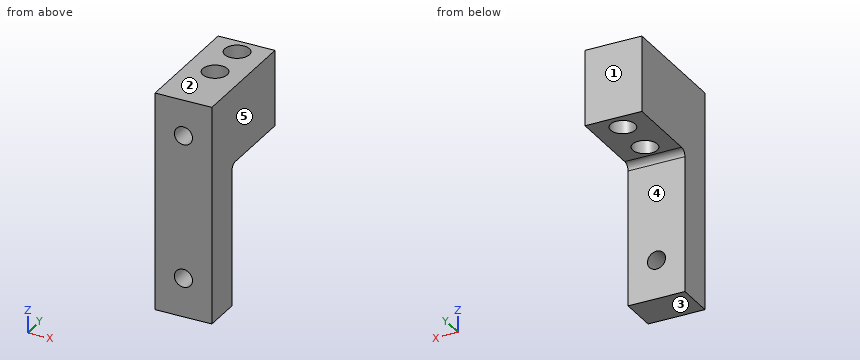
```python
from build123d import *

# Parameters (mm, degrees)
SKETCH1_W                 = 18.25
SKETCH1_H                 = 10
BOSS_EXTRUDE1_DEPTH       = 4.7625
F_1_64_TAPPED_HOLE1_D     = 1.5113
F_1_64_TAPPED_HOLE1_DEPTH = 3.5
F_1_64_TAPPED_HOLE1_TIP   = 0.454040327
SKETCH5_W                 = 11.9
SKETCH5_H                 = 6.825
CUT_EXTRUDE2_DEPTH        = 10
FILLET1_R                 = 0.5334
SKETCH2_R                 = 1.03
CUT_EXTRUDE1_DEPTH        = 20.512660153


with BuildPart() as part:
    # Sketch1 → Boss-Extrude1 (new body)
    with BuildSketch(Plane(origin=(0, 0, 0), x_dir=(0, 0, -1), z_dir=(1, 0, 0))):
        Rectangle(SKETCH1_W, SKETCH1_H)
    extrude(amount=BOSS_EXTRUDE1_DEPTH)

    # #1-64 Tapped Hole1
    with Locations(Plane(origin=(0, -5, 0), x_dir=(-1, 0, 0), z_dir=(0, -1, 0))):
        with Locations((-2.38125, -6.125), (-2.38125, 5.875)):
            Hole(F_1_64_TAPPED_HOLE1_D / 2, depth=F_1_64_TAPPED_HOLE1_DEPTH)
            with Locations((0, 0, -(F_1_64_TAPPED_HOLE1_DEPTH + F_1_64_TAPPED_HOLE1_TIP / 2))):  # 118° drill point
                Cone(0, F_1_64_TAPPED_HOLE1_D / 2, F_1_64_TAPPED_HOLE1_TIP, mode=Mode.SUBTRACT)

    # Sketch5 → Cut-Extrude2 (cut)
    with BuildSketch(Plane(origin=(4.7625, 0, 0), x_dir=(0, 0, -1), z_dir=(1, 0, 0))):
        with Locations((3.175, 1.5875)):
            Rectangle(SKETCH5_W, SKETCH5_H)
    extrude(amount=-CUT_EXTRUDE2_DEPTH, mode=Mode.SUBTRACT)

    # Fillet1
    fillet1_edges = [part.edges().sort_by_distance(p)[0] for p in [
        (2.38125, -1.825, 2.775),
    ]]
    fillet(fillet1_edges, radius=FILLET1_R)

    # Sketch2 → Cut-Extrude1 (cut, through all)
    with BuildSketch(Plane(origin=(0, 0, -9.125), x_dir=(-1, 0, 0), z_dir=(0, 0, -1))):
        with Locations((-2.38125, 3.5)):
            Circle(SKETCH2_R)
        with Locations((-2.38125, 0)):
            Circle(SKETCH2_R)
    extrude(amount=-CUT_EXTRUDE1_DEPTH, mode=Mode.SUBTRACT)


solid = part.part
```
Input: part model. Units: mm. Frame: model coordinates. Face numbers are marked on the shaded views. A direction names the side the tool comes from. Round coordinates to 2 decimals unless told otherwise and drop trailing zeros. Order: outer loops, then holes, each group sorted by start corner. A loop starts at its lowest first (then second) coordinate and runs counter-clockwise, first axis right, second up. Notation, with made-up numbers: (26.5, -12) - (45.5, -12) arc R6 ccw to (45.5, -6) - close; hole circle Ø6 at (0, -14.75). An arc over 180 degrees is marked (long way). One line per question, with ' | ' between items. Start each with the question number.
1) Ray query, probe 1 along Z at (x, y) = (2.5, -4) (3 decimals); probe 2 along Z at (x, y) = (4.3, 3) (3 decimals); probe 3 along Y at (x, z) = (1.45, 5.5). Return the intervals inside material, ascending.
2) Set-up query: the marked faces 4 and 5. Return all of +Z, -Z, +X, -X, +Y, -Y with unobstructed straight access to the full face (end or side cutting, diameter ignored); none if empty.
3) Pull-direction query (Z, two-part tool) for the marked faces 1, 2 and 3; classes: +Z half, -Z half, draft (parallel to the pull), parting line (faces both ways), or undercut.
4) Cut plane A-A, the plane y = 0.5. Return the cut outline in (x, z) (1 decimal).
5) Cut plane D-D, the plane y = -3.75. Return the cut outline in (x, z) (1 decimal).
6) Cut plane B-B, the plane x = 0.3. Return the cut outline in (y, z) (3 decimals), then the cut area to 3 significant figures.
7) Cut plane C-C, the plane z = 5. Return the cut outline in (x, y), then the cut area to 3 significant figures.
8) Contact query for a flat-ended pin moving along its axis: P1, Ø2.5, axis at x = 3.5, y = 3, coming from the -Z side (3 decimals). Output: stop coordinate, or through.
Worked out:
1) probe 1: z = -9.125 to -6.621, -5.129 to 5.379, 6.871 to 9.125 | probe 2: z = 2.775 to 9.125 | probe 3: y = -5 to -0.44, 0.44 to 3.06, 3.94 to 5
2) face 4: -Z, +X, -X, +Y | face 5: +Z, -Z, +X, +Y, -Y
3) face 1: draft | face 2: +Z half | face 3: -Z half
4) outline: (0, 2.8) - (1.5, 2.8) - (1.5, 9.1) - (0, 9.1) - close; (3.3, 2.8) - (4.8, 2.8) - (4.8, 9.1) - (3.3, 9.1) - close
5) outline: (0, -9.1) - (4.8, -9.1) - (4.8, 9.1) - (0, 9.1) - close; hole circle Ø1.5 at (2.4, -5.9); hole circle Ø1.5 at (2.4, 6.1)
6) outline: (-5, -9.125) - (-1.825, -9.125) - (-1.825, 2.242) arc R0.533 cw to (-1.292, 2.775) - (5, 2.775) - (5, 9.125) - (-5, 9.125) - close | area: 101 mm^2
7) outline: (0, -5) - (4.76, -5) - (4.76, 5) - (0, 5) - close; hole circle Ø2.06 at (2.38, 0); hole circle Ø2.06 at (2.38, 3.5) | area: 41.0 mm^2
8) P1: stops at z = 2.775
